from build123d import *

# Parameters (mm, degrees)
F0_R     = 38.0889
F0_R_2   = 1.4111
F0_R_3   = 1.1611
F1_DEPTH = 3.175


with BuildPart() as f1:
    # F0 (on Front) → F1 (new body)
    with BuildSketch(Plane.XZ):
        Circle(F0_R)
        with Locations((-24.395184, -24.395184)):
            Circle(F0_R_2, mode=Mode.SUBTRACT)
        with Locations((-7.778175, -7.778175)):
            Circle(F0_R_3, mode=Mode.SUBTRACT)
        with Locations((24.395184, -24.395184)):
            Circle(F0_R_2, mode=Mode.SUBTRACT)
        with Locations((7.778175, -7.778175)):
            Circle(F0_R_3, mode=Mode.SUBTRACT)
        with Locations((-7.778175, 7.778175)):
            Circle(F0_R_3, mode=Mode.SUBTRACT)
        with Locations((-24.395184, 24.395184)):
            Circle(F0_R_2, mode=Mode.SUBTRACT)
        with Locations((7.778175, 7.778175)):
            Circle(F0_R_3, mode=Mode.SUBTRACT)
        with Locations((24.395184, 24.395184)):
            Circle(F0_R_2, mode=Mode.SUBTRACT)
    extrude(amount=F1_DEPTH)


solid = f1.part
Check sheet for the modelled part. Datum: model origin and axes. Units: mm. Give positions to 0.01 mm unless a question says otherwise; leave off trailing zeros. Write each loop counter-clockwise with the first axis right and the second up, starting at its lowest first coordinate (ties: lowest second). Pieces come first, ordered by that corner, then holes. Notation, with made-up numbers: (20.5, 63.25) -> (25.5, 63.25) arc R12 ccw to (25.5, 75.25) -> close; hole circle Ø3 at (20.25, -10.5). An arc over 180 degrees is marked (long way). Use one line per item in the form item = value. Start each with the question number.
1. Section check A-A (y = -2.2). Count the separate pieces of the cut face and the enclosed holes in it, and give its area (3 significant figures).
2. Mould release check, pull along X, two halves, no side actions. Record for faces 1 (the flat face through (-1, 0, 1)), 2 (the cylindrical face through (-30.226, -1.565, -23.177)), 3 (the cylindrical face through (6.62, -1.57, 7.83)): pulls with the +X half, pulls with the -X half, needs draft (parallel to the pull), parting line crosses it, or undercut.
3. Thickness scan on line 1 along X through (y, z) = (-1.25, 7); line 2 along X through (y, z) = (-1.6, 25). Record the ranges inside material, lowest first. Write a range as from..to.
4. Go/stop test with flat-tipped pins: P1, Ø1.5, axis at x = -26.5, y = -1.5, coming from the -Z side; P2, Ø1, axis at x = -20, y = -1, coming from the -Z side. Record where each tip stops, or that it passes through.
5. Section check B-B (z = -21.5). Record the cut outline in (x, y) (3 decimals), and give its area (3 significant figures).
6. Section check C-C (x = -21). Record the cut outline in (y, z) (3 decimals), and give its area (3 significant figures).
Conclusion:
q1.separate_pieces = 1
q1.enclosed_holes = 8
q1.area = 4,520 mm²
q2.face_1 = needs draft
q2.face_2 = parting line crosses it
q2.face_3 = undercut
q3.line_1 = -37.44..-8.64, -6.92..6.92, 8.64..37.44
q3.line_2 = -28.74..-25.67, -23.12..23.12, 25.67..28.74
q4.P1 = -28.07
q4.P2 = -32.72
q5.outline = (-31.441, -3.175) -> (31.441, -3.175) -> (31.441, 0) -> (-31.441, 0) -> close
q5.area = 200 mm²
q6.outline = (-3.175, -31.777) -> (0, -31.777) -> (0, 31.777) -> (-3.175, 31.777) -> close
q6.area = 202 mm²
